The figure shows three views and two pictorial views of one solid part (mm, origin at its lowest corner). Answer the questions. Round coordinates to 2 decimals unless told otherwise and drop trailing zeros. Loops run counter-clockwise (first coordinate to the right, second up) from the corner with the lowest first, then second, coordinate; pieces in that order, holes last. Notation, with made-up numbers: (-20, -28) -> (20, -28) arc R20 cw to (20, -10) -> close; hole circle Ø1 at (9.5, 61.25). An arc over 180 degrees is marked (long way). Write each question's results on one line, items separated by ' | '. Start each with the question number.
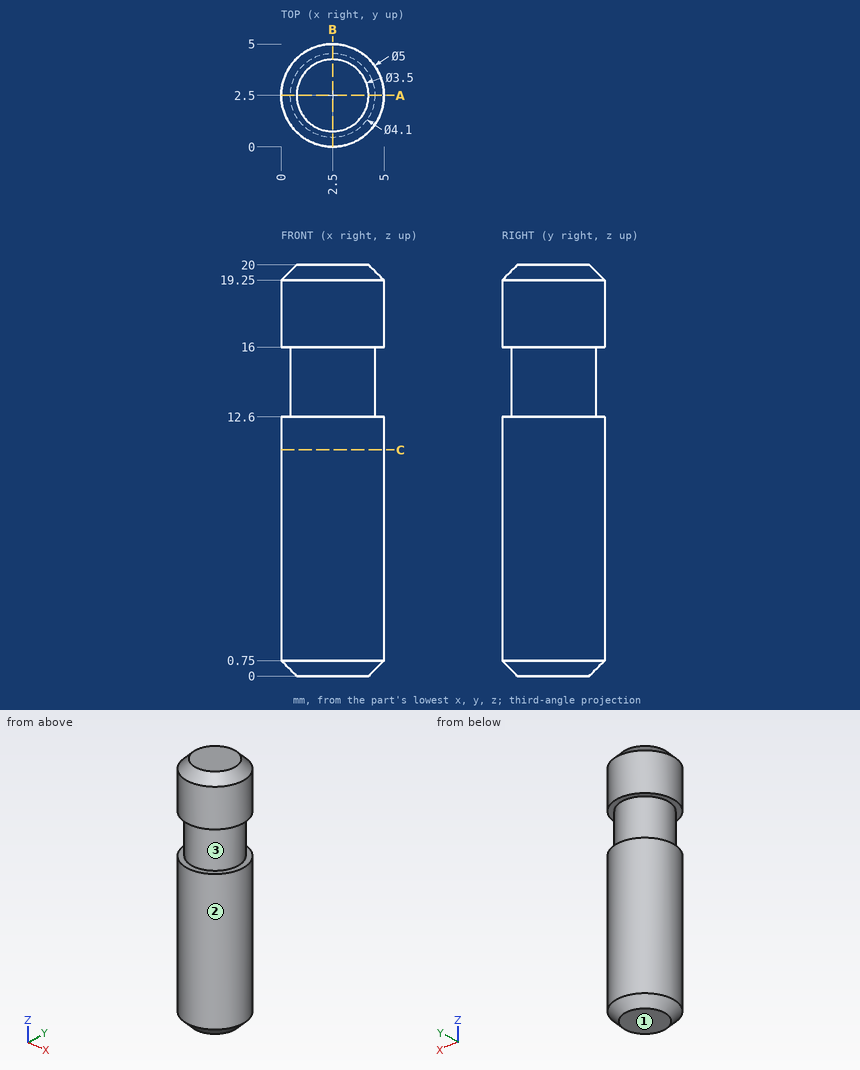
Item 1: The part is cut by section C-C, the plane z = 11. Give the vertices of the cut face in (x, y).
Item 2: Straight lines are drawn through the part: L1, parallel to X at y = 2.6, z = 1.75; L2, parallel to Z at x = 1.3, y = 0.55; L3, parallel to X at y = 0.6, z = 10.25. For each, find the intervals that lie inside material, in ascending order. Write a range as [from, to].
Item 3: This flat-tipped pin is pushed along its axis until it touches: pin 1 Ø3 at (x, z) = (3, 6.5) entering from +Y. Where does it stop, or does it pass through?
Item 4: The part is cut by section A-A, the plane y = 2.5. Give the vertices of the cut face in (x, z).
Item 5: Determine the mould class of the marked faces 1, 2 and 3 for opening direction Z: +Z half, -Z half, draft (parallel to the pull), parting line (faces both ways), or undercut.
Report:
1) outline: circle Ø5 at (2.5, 2.5)
2) L1: x = [0, 5] | L2: z = [0.54, 12.6], [16, 19.46] | L3: x = [0.88, 4.12]
3) pin 1: stops at y = 5
4) outline: (0, 0.75) -> (0.75, 0) -> (4.25, 0) -> (5, 0.75) -> (5, 12.6) -> (4.55, 12.6) -> (4.55, 16) -> (5, 16) -> (5, 19.25) -> (4.25, 20) -> (0.75, 20) -> (0, 19.25) -> (0, 16) -> (0.45, 16) -> (0.45, 12.6) -> (0, 12.6) -> close
5) face 1: -Z half | face 2: draft | face 3: undercut
